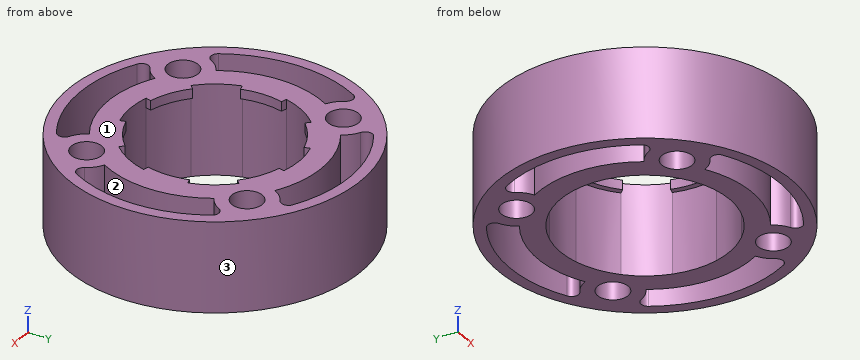
```python
from build123d import *

# Parameters (mm, degrees)
F0_R            = 20.6375
F0_R_2          = 2.15265
F1_DEPTH        = 12.7
F3_DEPTH        = 12.7
F4_COUNT        = 6
F4_ANGLE        = 300
F6_R            = 11.90625
F7_DEPTH        = 11.36015
F9_DEPTH        = 12.7
F9_COPIES_COUNT = 4
F10_R           = 1.0241935484


# Not quite as in the source:
# - a pattern or mirror of a feature is missing from the dataset's text; its kind, count and spacing are read off the source's solid


with BuildPart() as f1:
    # F0 (on Top) → F1 (new body)
    with BuildSketch(Plane.XY):
        Circle(F0_R)
        with Locations((-11.2253201513, -11.2253201513)):
            Circle(F0_R_2, mode=Mode.SUBTRACT)
        with Locations((11.2253201513, -11.2253201513)):
            Circle(F0_R_2, mode=Mode.SUBTRACT)
        with Locations((-11.2253201513, 11.2253201513)):
            Circle(F0_R_2, mode=Mode.SUBTRACT)
        with BuildLine():
            ThreePointArc((0, 11.1125), (7.8577241059, 7.8577241059), (11.1125, 0))
            ThreePointArc((11.1125, 0), (-7.8577241059, -7.8577241059), (0, 11.1125))
        make_face(mode=Mode.SUBTRACT)
        with Locations((11.2253201513, 11.2253201513)):
            Circle(F0_R_2, mode=Mode.SUBTRACT)
    extrude(amount=F1_DEPTH)

    # F2 (on face) → F3 (cut, through all)
    with BuildSketch(Plane.XY.offset(12.7)):
        with BuildLine():
            ThreePointArc((-2.8761266387, 10.7338507446), (0, 11.1125), (2.8761266387, 10.7338507446))
            Line((2.8761266387, 10.7338507446), (3.0815642558, 11.5005543693))
            ThreePointArc((3.0815642558, 11.5005543693), (0, 11.90625), (-3.0815642558, 11.5005543693))
            Line((-3.0815642558, 11.5005543693), (-2.8761266387, 10.7338507446))
        make_face()
    f3 = extrude(amount=-F3_DEPTH, mode=Mode.SUBTRACT)

    # F4: F3 ×6 about axis
    f4_axis = Axis((0, 0, 0), (0, 0, -1))
    for i in range(1, F4_COUNT):
        add(f3.rotate(f4_axis, i * F4_ANGLE / (F4_COUNT - 1)), mode=Mode.SUBTRACT)

    # F6 (on face) → F7 (cut, through all)
    with BuildSketch(Plane(origin=(0, 0, 0), x_dir=(1, 0, 0), z_dir=(0, 0, -1))):
        Circle(F6_R)
    extrude(amount=-F7_DEPTH, mode=Mode.SUBTRACT)

    # F8 (on face) → F9 (cut, through all)
    with BuildSketch(Plane(origin=(0, 0, 0), x_dir=(1, 0, 0), z_dir=(0, 0, -1))):
        with BuildLine():
            ThreePointArc((11.5039191556, -15.1842795042), (9.251826165, -14.6686177057), (7.6685282311, -12.9860608474))
            ThreePointArc((7.6685282311, -12.9860608474), (0, -15.08125), (-7.6685282311, -12.9860608474))
            ThreePointArc((-7.6685282311, -12.9860608474), (-9.251826165, -14.6686177057), (-11.5039191556, -15.1842795042))
            ThreePointArc((-11.5039191556, -15.1842795042), (0, -19.05), (11.5039191556, -15.1842795042))
        make_face()
    f9 = extrude(amount=-F9_DEPTH, mode=Mode.SUBTRACT)

    # F9_copies: F9 ×4 about axis
    f9_copies_axis = Axis((0, 0, 0), (0, 0, 1))
    for i in range(1, F9_COPIES_COUNT):
        add(f9.rotate(f9_copies_axis, i * 360 / F9_COPIES_COUNT), mode=Mode.SUBTRACT)

    # F10
    f10_edges = [f1.edges().sort_by_distance(p)[0] for p in [
        (-11.503919, 15.18428, 6.35),
        (11.503919, 15.18428, 6.35),
        (11.503919, -15.18428, 6.35),
        (-11.503919, -15.18428, 6.35),
        (-15.18428, -11.503919, 6.35),
        (-15.18428, 11.503919, 6.35),
        (15.18428, 11.503919, 6.35),
        (15.18428, -11.503919, 6.35),
    ]]
    fillet(f10_edges, radius=F10_R)


solid = f1.part
```
Here's how the part is built. I have some questions about the finished solid (model axes, mm). Face numbers are marked on the shaded views. Coordinates: 2 decimals unless noted, no trailing zeros. Write each loop counter-clockwise with the first axis right and the second up, starting at its lowest first coordinate (ties: lowest second). Pieces come first, ordered by that corner, then holes. Notation, with made-up numbers: (-35.5, 41.5) -> (-16.5, 41.5) arc R29 ccw to (-16.5, 65.5) -> close; hole circle Ø7 at (20, -7). An arc over 180 degrees is marked (long way). Use a Markdown table: item, result. Add a question column.
(1) Please list where these lines run through material, in increasing order: line 1 (X direction, y = 9.5, z = 10.75); line 2 (X direction, y = 9, z = 5.75); line 3 (Y direction, x = -5.5, z = 9.75).
(2) If we section it at B-B, the plane y = 6.5: Write out the boundary of the cut face in (x, z), and give its area (3 significant figures).
(3) If we section it at D-D, the plane z = 3.5: State how many separate pieces and enclosed holes the cut face has, and give its area (3 significant figures).
(4) I'm going to push flat-ended pins straight in: P1, Ø1.3, axis at x = -11, y = 1.5, coming from the -Z side; P2, Ø5, axis at x = 5.5, z = 10, coming from the -Y side; P3, Ø8, axis at x = -15, y = 9.5, coming from the -Z side; P4, Ø4, axis at x = -6.5, z = 1.5, coming from the +Y side. Where does each tip first touch, or does it pass through?
(5) If we section it at A-A, the plane x = 0: Write out the boundary of the cut face in (y, z).
(6) If we section it at C-C, the plane x = 7: Write out the boundary of the cut face in (y, z).
(7) We'd pull the mould along Y, two halves only. Please class the marked faces 1, 2 and 3: +Y half, -Y half, draft (parallel to the pull), parting line (faces both ways), or undercut.
Outcome:
| question | item | result |
|---|---|---|
| 1 | line 1 | x = -18.32 to -16.51, -14.81 to -12.51, -9.94 to -7.18, 7.18 to 9.94, 12.51 to 14.81, 16.51 to 18.32 |
| 1 | line 2 | x = -18.57 to -16.79, -14.51 to -7.79, 7.79 to 14.51, 16.79 to 18.57 |
| 1 | line 3 | y = -19.89 to -18.24, -14.04 to -10.56, 10.56 to 14.04, 18.24 to 19.89 |
| 2 | outline | (-19.59, 0) -> (-17.91, 0) -> (-17.91, 12.7) -> (-19.59, 12.7) -> close; (-13.61, 0) -> (-9.98, 0) -> (-9.98, 12.7) -> (-13.61, 12.7) -> close; (9.98, 0) -> (13.61, 0) -> (13.61, 12.7) -> (9.98, 12.7) -> close; (17.91, 0) -> (19.59, 0) -> (19.59, 12.7) -> (17.91, 12.7) -> close |
| 2 | area | 135 mm^2 |
| 3 | separate pieces | 1 |
| 3 | enclosed holes | 9 |
| 3 | area | 535 mm^2 |
| 4 | P1 | stops at z = 11.36 |
| 4 | P2 | stops at y = -20.42 |
| 4 | P3 | stops at z = 0 |
| 4 | P4 | stops at y = 20.14 |
| 5 | outline | (-20.64, 0) -> (-19.05, 0) -> (-19.05, 12.7) -> (-20.64, 12.7) -> close; (-15.08, 0) -> (-11.91, 0) -> (-11.91, 12.7) -> (-15.08, 12.7) -> close; (11.91, 0) -> (15.08, 0) -> (15.08, 12.7) -> (11.91, 12.7) -> close; (19.05, 0) -> (20.64, 0) -> (20.64, 12.7) -> (19.05, 12.7) -> close |
| 6 | outline | (-19.41, 0) -> (-17.72, 0) -> (-17.72, 12.7) -> (-19.41, 12.7) -> close; (-13.36, 0) -> (-9.63, 0) -> (-9.63, 11.36) -> (-8.63, 11.36) -> (-8.63, 12.7) -> (-13.36, 12.7) -> close; (8.63, 11.36) -> (9.63, 11.36) -> (9.63, 0) -> (13.36, 0) -> (13.36, 12.7) -> (8.63, 12.7) -> close; (17.72, 0) -> (19.41, 0) -> (19.41, 12.7) -> (17.72, 12.7) -> close |
| 7 | face 1 | draft |
| 7 | face 2 | undercut |
| 7 | face 3 | parting line |
